```python
from build123d import *

# Parameters (mm, degrees)
SKETCH1_R           = 2.4638
BOSS_EXTRUDE1_DEPTH = 4.445


with BuildPart() as part:
    # Sketch1 → Boss-Extrude1 (new body)
    with BuildSketch(Plane(origin=(0, 0, 0), x_dir=(1, 0, 0), z_dir=(0, 1, 0))):
        with BuildLine():
            ThreePointArc((5.6388, -31.75), (0, -37.3888), (-5.6388, -31.75))
            Line((-5.6388, -31.75), (-5.6388, -25.4))
            Line((-5.6388, -25.4), (-25.4, -25.4))
            Line((-25.4, -25.4), (-25.4, 25.4))
            Line((-25.4, 25.4), (-5.6388, 25.4))
            Line((-5.6388, 25.4), (-5.6388, 31.75))
            ThreePointArc((-5.6388, 31.75), (0, 37.3888), (5.6388, 31.75))
            Line((5.6388, 31.75), (5.6388, 25.4))
            Line((5.6388, 25.4), (25.4, 25.4))
            Line((25.4, 25.4), (25.4, -25.4))
            Line((25.4, -25.4), (5.6388, -25.4))
            Line((5.6388, -25.4), (5.6388, -31.75))
        make_face()
        with Locations(Location((0, 31.75, 0), (0, 0, 270))):
            Circle(SKETCH1_R, mode=Mode.SUBTRACT)
        with Locations(Location((0, -31.75, 0), (0, 0, 270))):
            Circle(SKETCH1_R, mode=Mode.SUBTRACT)
    extrude(amount=BOSS_EXTRUDE1_DEPTH)


solid = part.part
```
Part model, mm, in its own coordinate system. A direction names the side the tool comes from. Round coordinates to 2 decimals unless told otherwise and drop trailing zeros. Loops run counter-clockwise (first coordinate to the right, second up) from the corner with the lowest first, then second, coordinate; pieces in that order, holes last.
Item 1: Cut at C-C, the plane x = 15. Give the cut face in (y, z) (3 decimals), then the cut area to 3 significant figures.
Item 2: Cut at A-A, the plane x = 0. Give the cut face in (y, z) (3 decimals).
Item 3: Drop flat-ended pins along their axis: P1, Ø1, axis at x = 5, y = 1, coming from the +Z side; P2, Ø2, axis at x = 18.5, y = 1.5, coming from the +Z side; P3, Ø2, axis at y = 3.5, z = -27.5, coming from the -X side. Give the stop position or say it passes through.
Item 4: Cut at B-B, the plane y = 2. Give the cut face in (x, z), then the cut area to 3 significant figures.
Item 5: 3-axis set-ups, long thin cutter, end or side, ignore diameter. For faces 1 (the face through (-5.639, 2, -29)), 2 (the face through (5.639, 2, -29)), 3 (the face through (16, 2, 25.4)): which of +Z, -Z, +X, -X, +Y, -Y reach the whole face in a straight line?
Item 6: Drill centre lines: line 1 (X direction, y = 2.9, z = -31.75); line 2 (Z direction, x = -15.5, y = 0.35); line 3 (Z direction, x = 1.5, y = 1.8). Where is each one in solid material? Low to high.
Item 7: Mould opens along Z. For faces 4 (the face through (0.124, 2.191, 37.387)), 5 (the face through (0.74, 2.19, -29.4)), 6 (the face through (1, 2, 34)), 7 (the face through (5.639, 2, 29)) say: +Z half, -Z half, draft (parallel to the pull), parting line (faces both ways), or undercut.
A:
1. outline: (0, -25.4) - (4.445, -25.4) - (4.445, 25.4) - (0, 25.4) - close
1. area: 226 mm2
2. outline: (0, -37.389) - (4.445, -37.389) - (4.445, -34.214) - (0, -34.214) - close; (0, -29.286) - (4.445, -29.286) - (4.445, 29.286) - (0, 29.286) - close; (0, 34.214) - (4.445, 34.214) - (4.445, 37.389) - (0, 37.389) - close
3. P1: stops at z = 35.15
3. P2: stops at z = 25.4
3. P3: stops at x = -5.64
4. outline: (-25.4, -25.4) - (-5.64, -25.4) - (-5.64, -31.75) arc R5.64 ccw to (5.64, -31.75) - (5.64, -25.4) - (25.4, -25.4) - (25.4, 25.4) - (5.64, 25.4) - (5.64, 31.75) arc R5.64 ccw to (-5.64, 31.75) - (-5.64, 25.4) - (-25.4, 25.4) - close; hole circle Ø4.93 at (0, -31.75); hole circle Ø4.93 at (0, 31.75)
4. area: 2,790 mm2
5. face 1: -Z, -X, +Y, -Y
5. face 2: -Z, +X, +Y, -Y
5. face 3: +Z, +X, +Y, -Y
6. line 1: x = -5.64 to -2.46, 2.46 to 5.64
6. line 2: z = -25.4 to 25.4
6. line 3: z = -37.19 to -33.7, -29.8 to 29.8, 33.7 to 37.19
7. face 4: +Z half
7. face 5: undercut
7. face 6: undercut
7. face 7: draft
